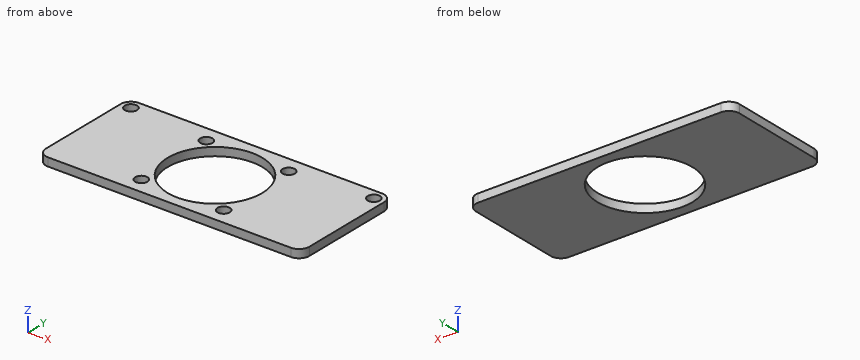
```python
from build123d import *

# Parameters (mm, degrees)
F0_R     = 1.5
F0_R_2   = 11.5
F1_DEPTH = 2
F2_DEPTH = 0.3


with BuildPart() as f1:
    # F0 (on Top) → F1 (new body)
    with BuildSketch(Plane.XY):
        with BuildLine():
            ThreePointArc((32, 11.5), (31.267767, 13.267767), (29.5, 14))
            Line((29.5, 14), (-29.5, 14))
            ThreePointArc((-29.5, 14), (-31.267767, 13.267767), (-32, 11.5))
            Line((-32, 11.5), (-32, -11.5))
            ThreePointArc((-32, -11.5), (-31.267767, -13.267767), (-29.5, -14))
            Line((-29.5, -14), (29.5, -14))
            ThreePointArc((29.5, -14), (31.267767, -13.267767), (32, -11.5))
            Line((32, -11.5), (32, 11.5))
        make_face()
        with Locations((-10, -10)):
            Circle(F0_R, mode=Mode.SUBTRACT)
        with Locations((10, -10)):
            Circle(F0_R, mode=Mode.SUBTRACT)
        with Locations((-29.5, 11.5)):
            Circle(F0_R, mode=Mode.SUBTRACT)
        with Locations((-10, 10)):
            Circle(F0_R, mode=Mode.SUBTRACT)
        Circle(F0_R_2, mode=Mode.SUBTRACT)
        with Locations((10, 10)):
            Circle(F0_R, mode=Mode.SUBTRACT)
        with Locations((29.5, 11.5)):
            Circle(F0_R, mode=Mode.SUBTRACT)
    extrude(amount=F1_DEPTH)

    # F0 (on Top) → F2 (join)
    with BuildSketch(Plane.XY):
        with Locations((-29.5, 11.5)):
            Circle(F0_R)
        with Locations((-10, 10)):
            Circle(F0_R)
        with Locations((10, 10)):
            Circle(F0_R)
        with Locations((29.5, 11.5)):
            Circle(F0_R)
        with Locations((10, -10)):
            Circle(F0_R)
        with Locations((-10, -10)):
            Circle(F0_R)
    extrude(amount=F2_DEPTH)


solid = f1.part
```
CAD build for the part. Positions are in the model's coordinates, mm. Round coordinates to 2 decimals unless told otherwise and drop trailing zeros. Order: outer loops, then holes, each group sorted by start corner. A loop starts at its lowest first (then second) coordinate and runs counter-clockwise, first axis right, second up.
Item 1: Probe line 1 along Y through (x, z) = (-29.5, 1.2); line 2 along X through (y, z) = (10.5, 1.65); line 3 along X through (y, z) = (-4.5, 0.85). List the from-to ranges inside material, lowest first.
Item 2: Saw through at A-A on z = 1.3. Write the cut outline in (x, y), then the cut area to 3 significant figures.
Item 3: Saw through at C-C on y = 0. Write the cut outline in (x, z), then the cut area to 3 significant figures.
Item 4: Saw through at B-B on x = 0. Write the cut outline in (y, z), then the cut area to 3 significant figures.
Item 5: Pin check, flat tip, straight feed: pin 1 (1.5 mm diameter, centred on x = -10, y = 10, fed in from +Z). Stop position of the tip, or through.
Item 6: Saw through at D-D on x = 10. Write the cut outline in (y, z), then the cut area to 3 significant figures.
Reported:
1. line 1: y = -14 to 10, 13 to 14
1. line 2: x = -32 to -30.62, -28.38 to -11.41, -8.59 to -4.69, 4.69 to 8.59, 11.41 to 28.38, 30.62 to 32
1. line 3: x = -32 to -10.58, 10.58 to 32
2. outline: (-32, -11.5) arc R2.5 ccw to (-29.5, -14) - (29.5, -14) arc R2.5 ccw to (32, -11.5) - (32, 11.5) arc R2.5 ccw to (29.5, 14) - (-29.5, 14) arc R2.5 ccw to (-32, 11.5) - close; hole circle Ø3 at (-29.5, 11.5); hole circle Ø3 at (-10, -10); hole circle Ø23 at (0, 0); hole circle Ø3 at (-10, 10); hole circle Ø3 at (10, -10); hole circle Ø3 at (10, 10); hole circle Ø3 at (29.5, 11.5)
2. area: 1,330 mm2
3. outline: (-32, 0) - (-11.5, 0) - (-11.5, 2) - (-32, 2) - close; (11.5, 0) - (32, 0) - (32, 2) - (11.5, 2) - close
3. area: 82.0 mm2
4. outline: (-14, 0) - (-11.5, 0) - (-11.5, 2) - (-14, 2) - close; (11.5, 0) - (14, 0) - (14, 2) - (11.5, 2) - close
4. area: 10.0 mm2
5. pin 1: stops at z = 0.3
6. outline: (-14, 0) - (-5.68, 0) - (-5.68, 2) - (-8.5, 2) - (-8.5, 0.3) - (-11.5, 0.3) - (-11.5, 2) - (-14, 2) - close; (5.68, 0) - (14, 0) - (14, 2) - (11.5, 2) - (11.5, 0.3) - (8.5, 0.3) - (8.5, 2) - (5.68, 2) - close
6. area: 23.1 mm2
